Part model, mm, in its own coordinate system. A direction names the side the tool comes from. Round coordinates to 2 decimals unless told otherwise and drop trailing zeros. Loops run counter-clockwise (first coordinate to the right, second up) from the corner with the lowest first, then second, coordinate; pieces in that order, holes last. Notation, with made-up numbers: M 49,0.25 L 95,0.25 A23 ccw 95,32.25 Z; hole C -30,3.25 d6. An arc over 180 degrees is marked long. Write each question's results on one line, items separated by ' | '.
from build123d import *

# Parameters (mm, degrees)
F0_R     = 2
F1_DEPTH = 7
F2_R     = 1
F3_DEPTH = 5
F4_R     = 1
F5_DEPTH = 5


with BuildPart() as f1:
    # F0 (on Front) → F1 (new body)
    with BuildSketch(Plane.XZ):
        Circle(F0_R)
    extrude(amount=F1_DEPTH)

    # F2 (on Front) → F3 (join)
    with BuildSketch(Plane.XZ):
        Circle(F2_R)
    extrude(amount=-F3_DEPTH)

    # F4 (on face) → F5 (cut)
    with BuildSketch(Plane.XZ.offset(7)):
        Circle(F4_R)
    extrude(amount=-F5_DEPTH, mode=Mode.SUBTRACT)


solid = f1.part
Item 1: Band-saw the part on C-C on y = -3. Give the cut face in (x, z), and give its area (3 significant figures).
Filled sheet:
outline: C 0,0 d4; hole C 0,0 d2 | area: 9.42 mm^2
Item 2: Two-plate mould, pull along X, no slides. Class faces 4 (the cylindrical face through (0, 2, -1)), 5 (the flat face through (0, 5, 0)), 6 (the flat face through (0, -2, 0)): +X half, -X half, draft (parallel to the pull), parting line (faces both ways), or undercut.
Filled sheet:
face 4: parting line | face 5: draft | face 6: undercut
Item 3: Band-saw the part on D-D on y = 2.25. Give the cut face in (x, z), and give its area (3 significant figures).
Filled sheet:
outline: C 0,0 d2 | area: 3.14 mm^2
Item 4: Band-saw the part on A-A on x = 0. Give the cut face in (y, z).
Filled sheet:
outline: M -7,-2 L 0,-2 L 0,-1 L 5,-1 L 5,1 L 0,1 L 0,2 L -7,2 L -7,1 L -2,1 L -2,-1 L -7,-1 Z
Item 5: Band-saw the part on B-B on z = 0. Give the cut face in (x, y).
Filled sheet:
outline: M -2,-7 L -1,-7 L -1,-2 L 1,-2 L 1,-7 L 2,-7 L 2,0 L 1,0 L 1,5 L -1,5 L -1,0 L -2,0 Z
Item 6: Which spindle directions (+Z, -Z, +X, -X, +Y, -Y) get a long thin tool onto all of the face, cutting with end or side? Do faces 1 (the flat face through (1, -7, -1)), 2 (the cylindrical face through (0, -5, -1)), 3 (the flat face through (1, 0, -1)). Say none if no direction does.
Filled sheet:
face 1: +Z, -Z, +X, -X, -Y | face 2: -Y | face 3: +Y
Item 7: Wall check: L1, parallel to Z at x = 0, y = -4.7; L2, parallel to Y at x = -0.35, z = 0.4; L3, parallel to Y at x = 0.95, z = 0.85. Give the ranges that are in metal, low to high.
Filled sheet:
L1: -2 to -1, 1 to 2 | L2: -2 to 5 | L3: -7 to 0
Item 8: Drop a flat-ended pin along its axis: P1, Ø0.6, axis at x = -0.5, z = 0, coming from the -Y side. Give the stop position or say it passes through.
Filled sheet:
P1: y = -2
